Read the model definition and answer for the solid it produces. Units are mm, in the model's axes. Face numbers are marked on the shaded views. A direction names the side the tool comes from. Give positions to 0.01 mm unless a question says otherwise; leave off trailing zeros. Loops run counter-clockwise (first coordinate to the right, second up) from the corner with the lowest first, then second, coordinate; pieces in that order, holes last. Notation, with made-up numbers: (44, 30) - (74, 30) arc R19 ccw to (74, 66) - close; hole circle Ø8 at (3.25, 50.25). An arc over 180 degrees is marked (long way). Use a Markdown table: item, result. Add a question column.
Item 1: A cutting plane is placed at B-B (z = -5). Determine the outline of the cut face in (x, y), plus the area to 3 significant figures.
Item 2: A cutting plane is placed at A-A (x = 0). Determine the outline of the cut face in (y, z).
Item 3: Each of these flat-tipped pins is pushed along its axis until it touches: P1, Ø1, axis at y = 12.5, z = -6, coming from the -X side; P2, Ø3, axis at x = -9, z = -2.5, coming from the +Y side; P3, Ø2, axis at x = 12, y = 9.5, coming from the -Z side; P4, Ø4, axis at y = 11, z = 0.5, coming from the -X side. Where does it stop, or does it pass through?
Item 4: For a pull along X with two mould halves and no side action, classify the marked faces 4, 5 and 6 as +X half, -X half, draft (parallel to the pull), parting line (faces both ways), or undercut.
Item 5: A cutting plane is placed at C-C (z = 0). Determine the outline of the cut face in (x, y).
Item 6: Consider probe 1 along X at (y, z) = (1.55, 0); probe 2 along Z at (x, y) = (11, 3.6); probe 3 along Y at (x, z) = (0, 1.5). Determine where each line is inside the solid, lowest interval first. Write a range as [from, to].
Item 7: Which of the six approach directions +Z, -Z, +X, -X, +Y, -Y give full straight-line access (tool end or side, diameter ignored) to the marked faces 1, 2 and 3?
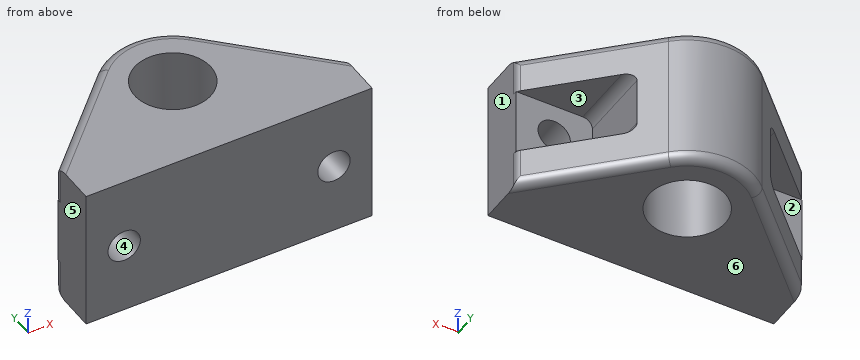
Autodesk Fusion 360 part; units mm, degrees
sketch "Sketch1" plane through (0, 0, 0) normal (0, 0, 1) x (1, 0, 0)
  line L0 (-15, 0) -> (15, 0)
  line L1 (15, 5) -> (4.9248, 14.9745)
  line L2 (-4.9248, 14.9745) -> (-15, 5)
  circle A0 centre (0, 10) radius 4
  line L3 (0, 2.5) -> (0, 20) construction
  arc A1 (4.9248, 14.9745) -> (-4.9248, 14.9745) centre (0, 10) ccw
  line L4 (15, 0) -> (15, 5)
  line L5 (-15, 0) -> (-15, 1)
  line L6 (-15, 1) -> (-15, 5)
  dimension "d1" = 8
  dimension "d2" = 7
  dimension "d3" = 10
  dimension "d4" = 30
  dimension "d5" = 5
extrude "Extrude1" add sketch "Sketch1" along normal mid plane 15
sketch "Sketch2" plane through (0, 0, 0) normal (0, 1, 0) x (1, 0, 0)
  line L0 (7, 3.5) -> (15, 3.5)
  line L1 (15, 3.5) -> (15, -3.5)
  line L2 (15, -3.5) -> (7, -3.5)
  line L3 (7, -3.5) -> (7, 3.5)
  line L4 (1.75, 0) -> (22.5, 0) construction
  line L5 (15, 7.5) -> (15, -7.5)
  point P0 (11, 0)
  dimension "d8" = 7
  dimension "d9" = 7
  dimension "d12" = 4
extrude "Extrude2" cut sketch "Sketch2" along normal through all from surface at 5
hole "Hole1" at (11, 0, 0) direction (0, 1, 0) diameter 3.4 end through all
mirror "Mirror1" about plane through (0, 0, 0) normal (1, 0, 0) of "Hole1", "Extrude2"
fillet "Fillet1" radius 1 14 edges at (7, 8.96, -3.5) (7, 8.96, 3.5) (-7, 8.96, -3.5) (-7, 8.96, 3.5) (9.9624, 9.9873, 7.5) (0, 17, 7.5) (-9.9624, 9.9873, 7.5) (-9.9624, 9.9873, -7.5) (0, 17, -7.5) (9.9624, 9.9873, -7.5) (15, 5, 5.5) (15, 5, -5.5) (-15, 5, -5.5) (-15, 5, 5.5)
Geometry says:
| question | item | result |
|---|---|---|
| 1 | outline | (-15, 0) - (15, 0) - (15, 4.58) arc R1 ccw to (14.7, 5.29) - (4.92, 14.97) arc R7 ccw to (-4.92, 14.97) - (-14.7, 5.29) arc R1 ccw to (-15, 4.58) - close; hole circle Ø8 at (0, 10) |
| 1 | area | 312 mm² |
| 2 | outline | (0, -7.5) - (6, -7.5) - (6, 7.5) - (0, 7.5) - close; (14, -7.5) - (16, -7.5) arc R1 ccw to (17, -6.5) - (17, 6.5) arc R1 ccw to (16, 7.5) - (14, 7.5) - close |
| 3 | P1 | x = -7.93 |
| 3 | P2 | y = 12.05 |
| 3 | P3 | through |
| 3 | P4 | x = -7 |
| 4 | face 4 | undercut |
| 4 | face 5 | -X half |
| 4 | face 6 | draft |
| 5 | outline | (-15, 0) - (-12.7, 0) - (-12.7, 5) - (-15, 5) - close; (-9.3, 0) - (9.3, 0) - (9.3, 5) - (7, 5) - (7, 12.92) - (4.92, 14.97) arc R7 ccw to (-4.92, 14.97) - (-7, 12.92) - (-7, 5) - (-9.3, 5) - close; (12.7, 0) - (15, 0) - (15, 5) - (12.7, 5) - close; hole circle Ø8 at (0, 10) |
| 6 | probe 1 | [-15, -12.7], [-9.3, 9.3], [12.7, 15] |
| 6 | probe 2 | [-7.5, -1.7], [1.7, 7.5] |
| 6 | probe 3 | [0, 6], [14, 17] |
| 7 | face 1 | +Z, -Z, +X, +Y, -Y |
| 7 | face 2 | -X, +Y |
| 7 | face 3 | +X, +Y |
